from build123d import *

# Parameters (mm, degrees)
F2_R     = 1.25
F3_DEPTH = 25


with BuildPart() as f1:
    # F0 (on Front) → F1 (revolve)
    with BuildSketch(Plane.XZ):
        Polygon((9, 9), (9, 0), (13.5, 0), (13.5, 1.525), (10.5, 1.525), (10.5, 2.525), (13.5, 2.525), (13.5, 4.05), (10.5, 4.05), (10.5, 4.716667), (13.5, 4.716667), (13.5, 6.241667), (10.5, 6.241667), (10.5, 6.908333), (13.5, 6.908333), (13.5, 8.433333), (10.5, 8.433333), (10.5, 9.1), (13.5, 9.1), (13.5, 10.5), (10, 10.5), (10, 9), align=None)
    revolve(axis=Axis((0, 0, 1e-06), (0, 0, -1)))

    # F2 (on face) → F3 (cut)
    with BuildSketch(Plane.XY.offset(10.5)):
        with Locations((0, 11.5)):
            Circle(F2_R)
        with Locations((-9.959292, 5.75)):
            Circle(F2_R)
        with Locations((-9.959292, -5.75)):
            Circle(F2_R)
        with Locations((0, -11.5)):
            Circle(F2_R)
        with Locations((9.959292, -5.75)):
            Circle(F2_R)
        with Locations((9.959292, 5.75)):
            Circle(F2_R)
    extrude(amount=-F3_DEPTH, mode=Mode.SUBTRACT)


solid = f1.part
Verification items for the finished model (mm, model axes). A direction names the side the tool comes from. Give positions to 0.01 mm unless a question says otherwise; leave off trailing zeros. Loops run counter-clockwise (first coordinate to the right, second up) from the corner with the lowest first, then second, coordinate; pieces in that order, holes last.
1) Sectioned sample at B-B, the plane x = 0. Count the separate pieces of the cut face and the enclosed holes in it, then the cut area to 3 significant figures.
2) Draft check along Z on faces 1 (the flat face through (-9, 3, 0)), 2 (the cylindrical face through (-5.192, -9.127, 8.771)), 3 (the cylindrical face through (-5.192, -9.127, 4.388)), 4 (the cylindrical face through (-2.93, 13.18, 0.77)). Enter one of: pulls with the +Z half, pulls with the -Z half, needs draft (parallel to the pull), parting line crosses it, or undercut.
3) Set-up check for faces 5 (the cylindrical face through (-5.192, -9.127, 2.032)), 6 (the flat face through (8.1, -7.1, 9.1)), 7 (the cylindrical face through (-10.5, -0.1, 6.6)), 8 (the cylindrical face through (5.192, 9.127, 2.032)): record each of +Z, -Z, +X, -X, +Y, -Y from which the full face is reachable in a straight line by a thin tool's end or side.
4) Thickness scan on line 1 along Z through (x, y) = (-2, 10.75) (3 decimals); line 2 along X through (y, z) = (-0.25, 0.5); line 3 along Y through (x, z) = (0, 6.5). Record the ranges inside material, lowest first.
5) Sectioned sample at C-C, the plane z = 9.75. Enter the section's corners in (x, y), then the cut area to 3 significant figures.
6) Sectioned sample at A-A, the plane z = 3. Enter the section's corners in (x, y), then the cut area to 3 significant figures.
7) Depth check by flat-ended pin: pin 1 Ø3 at (y, z) = (-8, 9) entering from -X; pin 2 Ø2 at (x, y) = (0, -11.5) entering from -Z; pin 3 Ø1 at (y, z) = (4, 3) entering from +X; pin 4 Ø2 at (x, z) = (8, 2.5) entering from -Y. Enter the tip coordinate at first touch or a pass-through.
Answers:
1. separate pieces: 12
1. enclosed holes: 0
1. area: 34.5 mm2
2. face 1: pulls with the -Z half
2. face 2: undercut
2. face 3: undercut
2. face 4: needs draft
3. face 5: -X, -Y
3. face 6: none
3. face 7: -X
3. face 8: +X, +Y
4. line 1: z = 0 to 1.525, 2.525 to 4.05, 4.717 to 6.242, 6.908 to 8.433, 9.1 to 10.5
4. line 2: x = -13.5 to -9, 9 to 13.5
4. line 3: y = -10.25 to -9, 9 to 10.25
5. outline: circle Ø27 at (0, 0); hole circle Ø2.5 at (-9.96, -5.75); hole circle Ø2.5 at (-9.96, 5.75); hole circle Ø20 at (0, 0); hole circle Ø2.5 at (0, -11.5); hole circle Ø2.5 at (0, 11.5); hole circle Ø2.5 at (9.96, -5.75); hole circle Ø2.5 at (9.96, 5.75)
5. area: 229 mm2
6. outline: circle Ø27 at (0, 0); hole circle Ø2.5 at (-9.96, -5.75); hole circle Ø2.5 at (-9.96, 5.75); hole circle Ø18 at (0, 0); hole circle Ø2.5 at (0, -11.5); hole circle Ø2.5 at (0, 11.5); hole circle Ø2.5 at (9.96, -5.75); hole circle Ø2.5 at (9.96, 5.75)
6. area: 289 mm2
7. pin 1: stops at x = -11.83
7. pin 2: passes through
7. pin 3: stops at x = 13.04
7. pin 4: stops at y = -11.54
